For this review, take the finished solid that the model builds, in its own axes (mm). Face numbers are marked on the shaded views. A direction names the side the tool comes from. Coordinates: 2 decimals unless noted, no trailing zeros. Loops run counter-clockwise (first coordinate to the right, second up) from the corner with the lowest first, then second, coordinate; pieces in that order, holes last. Notation, with made-up numbers: (26, -20) - (44, -20) arc R19 ccw to (44, 10) - close; hole circle Ø3 at (-5.75, 83.5). An arc over 180 degrees is marked (long way). Answer as a JSON object with one key per item and string values. Group by question number.
Item 1: We need section D-D (y = 12). Give the boundary of the cut face in (x, z), then the cut area to 3 significant figures.
Item 2: Tool access review of the marked faces 4, 5, 6, 7 and 8: name each direction out of +Z, -Z, +X, -X, +Y, -Y from which nothing blocks a thin tool from reaching the whole face with its end or side.
Item 3: Clearance check with flat-ended pins moving along their axes: pin 1 (14 mm diameter, centred on x = 0.5, y = -115.5, fed in from -Z); pin 2 (5 mm diameter, centred on x = -6.5, z = -9, fed in from -Y); pin 3 (9 mm diameter, centred on y = 12.5, z = 23.5, fed in from -X). State where each tip first meets the part, or that it passes through.
Item 4: We need section C-C (y = -34.5). Give the boundary of the cut face in (x, z), then the cut area to 3 significant figures.
Item 5: We need section B-B (x = 0). Give the boundary of the cut face in (y, z).
Item 6: We need section A-A (z = 40.5). Give the boundary of the cut face in (x, y), then the cut area to 3 significant figures.
Item 7: To check wall thickness, follow line 1 (X direction, y = 27.75, z = 30); line 2 (Z direction, x = -18, y = 25.75); line 3 (Y direction, x = 0, z = 6). State the ranges of each line that lie inside material, in increasing order.
Item 8: Mouldability with a two-part tool opening along Y and no side actions: class the marked faces 1, 2 and 3 as released by +Y, released by -Y, zero draft, split by the parting line, or undercut.
Autodesk Inventor part; units mm, degrees
ref_plane "YZ Plane" through (0, 0, 0) normal (1, 0, 0) x (0, 1, 0)
ref_plane "XZ Plane" through (0, 0, 0) normal (0, 1, 0) x (-1, 0, 0)
ref_plane "XY Plane" through (0, 0, 0) normal (0, 0, 1) x (1, 0, 0)
sketch "Sketch1" plane through (0, 0, 0) normal (0, 0, 1) x (1, 0, 0)
  line L0 (-30, 37.5) -> (30, 37.5)
  line L1 (30, 37.5) -> (30, -37.5)
  line L2 (30, -37.5) -> (-30, -37.5)
  line L3 (-30, -37.5) -> (-30, 37.5)
  line L4 (-30, 37.5) -> (30, -37.5) construction
  line L5 (30, 37.5) -> (-30, -37.5) construction
  circle A0 centre (0, -37.5) radius 30
  circle A1 centre (0, -37.5) radius 20
  circle A2 centre (0, -112.5) radius 23
  circle A3 centre (0, -112.5) radius 10
  line L6 (-23, -112.5) -> (-23, -56.7614)
  line L7 (23, -112.5) -> (23, -56.7614)
  line L8 (-30, 37.5) -> (30, 37.5)
  line L9 (30, 37.5) -> (30, 22.5)
  line L10 (30, 22.5) -> (-30, 22.5)
  line L11 (-30, 22.5) -> (-30, 37.5)
  line L12 (-5, 22.5) -> (5, 22.5)
  line L13 (5, 22.5) -> (5, -7.9196)
  line L14 (-5, -7.9196) -> (-5, 22.5)
  point P0 (0, 0)
  dimension "d0" = 60
  dimension "d1" = 75
  dimension "d2" = 60
  dimension "d3" = 40
  dimension "d4" = 46
  dimension "d5" = 20
  dimension "d6" = 75
  dimension "d7" = 15
  dimension "d9" = 25
extrude "Extrusion1" add sketch "Sketch1" along normal blind 15 contours L10 L14 A0 L3 | L1 A0 L13 L10 | A0 L7 A2 L6 | A2
extrude "Extrusion2" add sketch "Sketch1" along normal blind 45 contours L0 L1 L10 L3 | L10 L13 A0 L14
extrude "Extrusion3" add sketch "Sketch1" along normal blind 45 and the other way blind 15 contours A0 L2 A1 | L2 A1 A0
sketch "Sketch2" plane through (-30, 22.5, 15) normal (0, -1, 0) x (1, 0, 0)
  point P0 (30, -15)
sketch "Sketch3" plane through (-30, 22.5, 15) normal (0, -1, 0) x (1, 0, 0)
  point P0 (30, -15)
sketch "Sketch4" plane through (-30, 37.5, 0) normal (0, 1, 0) x (1, 0, 0)
  circle A0 centre (12, -30) radius 8
  line L0 (0, 0) -> (0, -45)
  line L1 (60, -45) -> (0, -45)
  circle A1 centre (48, -30) radius 8
  point P0 (30, 0)
  dimension "d18" = 16
  dimension "d19" = 12
  dimension "d20" = 15
extrude "Extrusion4" cut sketch "Sketch4" against normal blind 15
properties part number "cad@71"
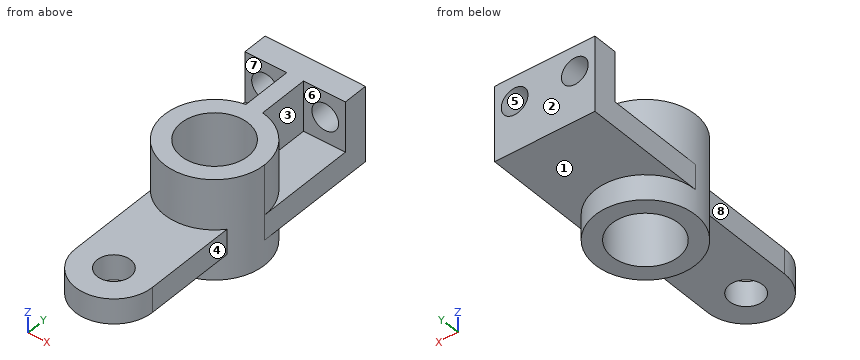
Check sheet entries:
{
 "1": {"outline": "(-30, 0) - (30, 0) - (30, 15) - (5, 15) - (5, 45) - (-5, 45) - (-5, 15) - (-30, 15) - close", "area": "1,200 mm2"},
 "2": {"face 4": "+Z, -Z, +X, -Y", "face 5": "+Y", "face 6": "+Z, +X", "face 7": "+Z, -X", "face 8": "+Z, -Z, -X, -Y"},
 "3": {"pin 1": "stops at z = 0", "pin 2": "stops at y = -67.23", "pin 3": "stops at x = -5"},
 "4": {"outline": "(-30, 0) - (-29.85, 0) - (-29.85, -15) - (-19.77, -15) - (-19.77, 45) - (-29.85, 45) - (-29.85, 15) - (-30, 15) - close; (19.77, -15) - (29.85, -15) - (29.85, 0) - (30, 0) - (30, 15) - (29.85, 15) - (29.85, 45) - (19.77, 45) - close", "area": "1,210 mm2"},
 "5": {"outline": "(-135.5, 0) - (-122.5, 0) - (-122.5, 15) - (-135.5, 15) - close; (-102.5, 0) - (-67.5, 0) - (-67.5, -15) - (-57.5, -15) - (-57.5, 45) - (-67.5, 45) - (-67.5, 15) - (-102.5, 15) - close; (-17.5, -15) - (-7.5, -15) - (-7.5, 0) - (37.5, 0) - (37.5, 45) - (-17.5, 45) - close"},
 "6": {"outline": "(-30, 22.5) - (-5, 22.5) - (-5, -7.92) arc R30 ccw (long way) to (5, -7.92) - (5, 22.5) - (30, 22.5) - (30, 37.5) - (-30, 37.5) - close; hole circle Ø40 at (0, -37.5)", "area": "2,770 mm2"},
 "7": {"line 1": "x = -30 to -26, -10 to 10, 26 to 30", "line 2": "z = 0 to 22, 38 to 45", "line 3": "y = -135.5 to -122.5, -102.5 to -57.5, -17.5 to 37.5"},
 "8": {"face 1": "zero draft", "face 2": "released by +Y", "face 3": "undercut"}
}
